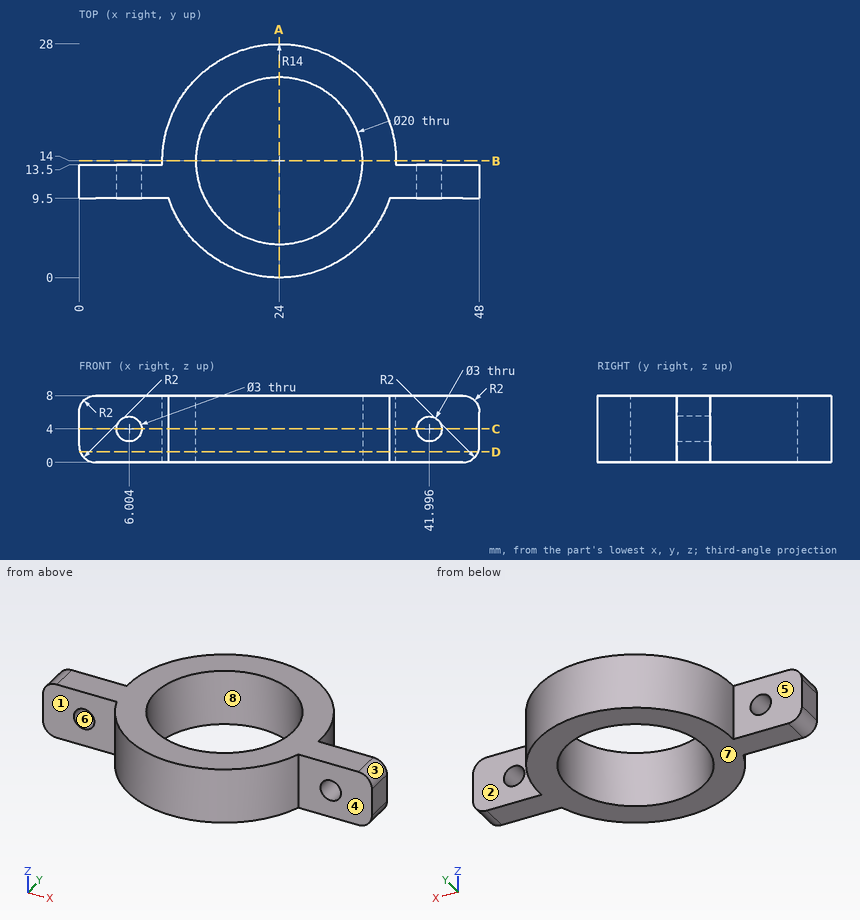
Check sheet for the drawn part. Datum: minimum x, y, z corner. Units: mm. A direction names the side the tool comes from. Give positions to 0.01 mm unless a question says otherwise; leave off trailing zeros. Order: outer loops, then holes, each group sorted by start corner. A loop starts at its lowest first (then second) coordinate and runs counter-clockwise, first axis right, second up. Notation, with made-up numbers: (59.5, -4.5) - (79.5, -4.5) arc R35 cw to (79.5, 29.5) - close; hole circle Ø2 at (21.25, 37). An arc over 180 degrees is marked (long way). Write item = value, one per line. Start each with the question number.
1) Gauge pin test, flat ends, axial feed: pin 1 Ø2.5 at (x, z) = (41.5, 5.5) entering from +Y; pin 2 Ø5 at (x, y) = (30, 10.5) entering from +Z (3 decimals); pin 3 Ø2.5 at (x, z) = (42.5, 3.5) entering from -Y; pin 4 Ø1.5 at (x, z) = (36.5, 6.5) entering from +Y. Record the tip position at first contact, or that the pin passes through.
2) Section check D-D (z = 1.25). Enter the section's corners in (x, y).
3) Section check B-B (y = 14). Enter the section's corners in (x, z).
4) Scan lines: L1, parallel to X at y = 12.5, z = 4 (1 decimal); L2, parallel to X at y = 10.4, z = 4 (1 decimal); L3, parallel to X at y = 5, z = 4.25 (1 decimal). Record each from-to range of solid material in increasing order.
5) Section check C-C (z = 4). Enter the section's corners in (x, y) (1 decimal), then the cut area to 3 significant figures.
6) Section check A-A (x = 24). Enter the section's corners in (y, z), then the cut area to 3 significant figures.
7) Draft check along Z on the marked faces 6, 7 and 8. Enter one of: released by +Z, released by -Z, zero draft, split by the parting line, or undercut.
8) Access from +Z, -Z, +X, -X, +Y, -Y to the whole of each face (thin tool, end or side, straight path). Record for the marked faces 1, 2, 3, 4 and 5.
Geometry check:
q1.pin_1 = 13.5
q1.pin_2 = through
q1.pin_3 = 9.5
q1.pin_4 = 21.61
q2.outline = (0.15, 9.5) - (10.74, 9.5) arc R14 ccw to (37.26, 9.5) - (47.85, 9.5) - (47.85, 13.5) - (37.99, 13.5) arc R14 ccw (long way) to (10.01, 13.5) - (0.15, 13.5) - close; hole circle Ø20 at (24, 14)
q3.outline = (10, 0) - (14, 0) - (14, 8) - (10, 8) - close; (34, 0) - (38, 0) - (38, 8) - (34, 8) - close
q4.L1 = 0 to 4.5, 7.5 to 14.1, 33.9 to 40.5, 43.5 to 48
q4.L2 = 0 to 4.5, 7.5 to 14.7, 33.3 to 40.5, 43.5 to 48
q4.L3 = 13.3 to 19.6, 28.4 to 34.7
q5.outline = (0, 9.5) - (4.5, 9.5) - (4.5, 13.5) - (0, 13.5) - close; (7.5, 9.5) - (10.7, 9.5) arc R14 ccw to (37.3, 9.5) - (40.5, 9.5) - (40.5, 13.5) - (38, 13.5) arc R14 ccw (long way) to (10, 13.5) - (7.5, 13.5) - close; (43.5, 9.5) - (48, 9.5) - (48, 13.5) - (43.5, 13.5) - close; hole circle Ø20 at (24, 14)
q5.area = 360 mm2
q6.outline = (0, 0) - (4, 0) - (4, 8) - (0, 8) - close; (24, 0) - (28, 0) - (28, 8) - (24, 8) - close
q6.area = 64.0 mm2
q7.face_6 = undercut
q7.face_7 = released by -Z
q7.face_8 = zero draft
q8.face_1 = +Z, -Z, -X, -Y
q8.face_2 = +Z, -Z, +X, +Y
q8.face_3 = +Z, +X, +Y, -Y
q8.face_4 = +Z, -Z, +X, -Y
q8.face_5 = +Z, -Z, -X, +Y
